Source: CAD feature listing. Evaluate the final solid. Frame: model axes, mm. Coordinates: 2 decimals unless noted, no trailing zeros. Write each loop counter-clockwise with the first axis right and the second up, starting at its lowest first coordinate (ties: lowest second). Pieces come first, ordered by that corner, then holes. Notation, with made-up numbers: M 27,-34 L 49,-34 A23 ccw 49,-14 Z; hole C -24,86 d2. An arc over 180 degrees is marked long. Write item = value, one per line. Start each with the question number.
1. Pin query (flat end, axial travel): pin 1 Ø8 at (x, y) = (102.5, -15) entering from -Z; pin 2 Ø1 at (y, z) = (-23.5, 1.5) entering from -X. Return the tip coordinate at first contact, or that it passes through.
2. Line query: line 1 along Y through (x, z) = (102.5, 0.95); line 2 along X through (y, z) = (-11.5, 2); line 3 along Y through (x, z) = (5, 1.1). Output: solid intervals per line, ascending.
3. Section query C-C (z = 1.75). Output: boundary loops of the cut face in (x, y).
4. Section query A-A (x = 27.5). Output: boundary loops of the cut face in (y, z).
5. Section query D-D (x = 5). Output: boundary loops of the cut face in (y, z), then the cut area to 3 significant figures.
6. Pull-direction query (X, two-part tool) for faces 1 (the face through (23.5, -18, 1.5)), 2 (the face through (116.99, -2.85, 1.52)), 3 (the face through (59, 0, 1)); classes: pulls with the +X half, pulls with the -X half, needs draft (parallel to the pull), parting line crosses it, or undercut.
7. Section query B-B (y = -15). Output: boundary loops of the cut face in (x, z).
```python
from build123d import *

# Parameters (mm, degrees)
ESQUISSE1_W             = 120
ESQUISSE1_H             = 30
ESQUISSE1_R             = 2
BOSS_EXTRU_1_DEPTH      = 3
CONG_1_R                = 10
ESQUISSE2_R             = 5
ENL_V_MAT_EXTRU_1_DEPTH = 3


with BuildPart() as part:
    # Esquisse1 → Boss.-Extru.1 (new body)
    with BuildSketch(Plane.XY):
        with Locations((60, -15)):
            Rectangle(ESQUISSE1_W, ESQUISSE1_H)
        with Locations((115, -15)):
            Circle(ESQUISSE1_R, mode=Mode.SUBTRACT)
        with Locations((5, -15)):
            Circle(ESQUISSE1_R, mode=Mode.SUBTRACT)
    extrude(amount=BOSS_EXTRU_1_DEPTH)

    # Congé1
    cong_1_edges = [part.edges().sort_by_distance(p)[0] for p in [
        (0, 0, 1.5),
        (120, 0, 1.5),
        (120, -30, 1.5),
        (0, -30, 1.5),
    ]]
    fillet(cong_1_edges, radius=CONG_1_R)

    # Esquisse2 → Enlèv. mat.-Extru.1 (cut)
    with BuildSketch(Plane.XY.offset(3)):
        with Locations((27.5, -15)):
            Circle(ESQUISSE2_R)
        with Locations((102.5, -15)):
            Circle(ESQUISSE2_R)
    extrude(amount=-ENL_V_MAT_EXTRU_1_DEPTH, mode=Mode.SUBTRACT)


solid = part.part
```
Results are:
q1.pin_1 = through
q1.pin_2 = 0.46
q2.line_1 = -30 to -20, -10 to 0
q2.line_2 = 0 to 23.93, 31.07 to 98.93, 106.07 to 120
q2.line_3 = -28.66 to -17, -13 to -1.34
q3.outline = M 0,-20 A10 ccw 10,-30 L 110,-30 A10 ccw 120,-20 L 120,-10 A10 ccw 110,0 L 10,0 A10 ccw 0,-10 Z; hole C 5,-15 d4; hole C 27.5,-15 d10; hole C 102.5,-15 d10; hole C 115,-15 d4
q4.outline = M -30,0 L -20,0 L -20,3 L -30,3 Z; M -10,0 L 0,0 L 0,3 L -10,3 Z
q5.outline = M -28.66,0 L -17,0 L -17,3 L -28.66,3 Z; M -13,0 L -1.34,0 L -1.34,3 L -13,3 Z
q5.area = 70.0 mm^2
q6.face_1 = undercut
q6.face_2 = pulls with the +X half
q6.face_3 = needs draft
q7.outline = M 0,0 L 3,0 L 3,3 L 0,3 Z; M 7,0 L 22.5,0 L 22.5,3 L 7,3 Z; M 32.5,0 L 97.5,0 L 97.5,3 L 32.5,3 Z; M 107.5,0 L 113,0 L 113,3 L 107.5,3 Z; M 117,0 L 120,0 L 120,3 L 117,3 Z
